Build history of the part. All positions in model axes, mm. A direction names the side the tool comes from. Round coordinates to 2 decimals unless told otherwise and drop trailing zeros. Loops run counter-clockwise (first coordinate to the right, second up) from the corner with the lowest first, then second, coordinate; pieces in that order, holes last. Notation, with made-up numbers: M 25.5,4.25 L 46.5,4.25 A5 ccw 46.5,10.25 Z; hole C 58,-40 d9. An arc over 180 degrees is marked long. Write each question's results on one line, items separated by ' | '. Start each with the question number.
```python
from build123d import *

# Parameters (mm, degrees)
F0_W     = 203.2
F0_H     = 208.396926
F1_DEPTH = 25.4
F2_R     = 25.4
F3_DEPTH = 25.4
F4_R     = 25.4
F5_DEPTH = 25.4


with BuildPart() as f1:
    # F0 (on Top) → F1 (new body)
    with BuildSketch(Plane.XY):
        Rectangle(F0_W, F0_H)
    extrude(amount=F1_DEPTH)

    # F2 (on face) → F3 (join)
    with BuildSketch(Plane.XY.offset(25.4)):
        with Locations((0, 63.5)):
            Circle(F2_R)
    extrude(amount=F3_DEPTH)

    # F4 (on face) → F5 (join, through all)
    with BuildSketch(Plane.XY.offset(25.4)):
        with Locations((0, -70.358)):
            Circle(F4_R)
    extrude(amount=F5_DEPTH)


solid = f1.part
```
Item 1: Saw through at A-A, the plane y = 63.5. Give the cut face in (x, z), then the cut area to 3 significant figures.
Item 2: Drill centre lines: line 1 along Y through (x, z) = (0.5, 39); line 2 along Z through (x, y) = (18.5, 6.5); line 3 along X through (y, z) = (-69, 43.5). Where is each one in solid material? Low to high. Write a range as [from, to].
Item 3: Saw through at B-B, the plane x = 0. Give the cut face in (y, z), then the cut area to 3 significant figures.
Item 4: Saw through at C-C, the plane z = 33.5. Give the cut face in (x, y), then the cut area to 3 significant figures.
Item 5: Drop flat-ended pins along their axis: pin 1 (1 mm diameter, centred on y = 51, z = 34.5, fed in from +X); pin 2 (12 mm diameter, centred on x = -69.5, y = -80, fed in from +Z). Give the stop position or say it passes through.
Item 6: Tool access for faces 5 (the flat face through (0, -70, 50.8)), 6 (the flat face through (-1, 1, 25.4)): list every direction of +Z, -Z, +X, -X, +Y, -Y with a clear straight run to the whole face (end or side of a thin tool).
Item 7: Saw through at D-D, the plane y = -74. Give the cut face in (x, z), then the cut area to 3 significant figures.
Item 8: Mould opens along Y. For faces 1 (the flat face through (-1, 1, 0)), 2 (the cylindrical face through (-5.506, -95.154, 37.922)), 3 (the cylindrical face through (-5.506, 38.704, 37.922)), 4 (the flat face through (-1, -104.198, 13)) say: released by +Y, released by -Y, zero draft, split by the parting line, or undercut.
Working result:
1) outline: M -101.6,0 L 101.6,0 L 101.6,25.4 L 25.4,25.4 L 25.4,50.8 L -25.4,50.8 L -25.4,25.4 L -101.6,25.4 Z | area: 6,450 mm²
2) line 1: y = [-95.75, -44.96], [38.1, 88.9] | line 2: z = [0, 25.4] | line 3: x = [-25.36, 25.36]
3) outline: M -104.2,0 L 104.2,0 L 104.2,25.4 L 88.9,25.4 L 88.9,50.8 L 38.1,50.8 L 38.1,25.4 L -44.96,25.4 L -44.96,50.8 L -95.76,50.8 L -95.76,25.4 L -104.2,25.4 Z | area: 7,870 mm²
4) outline: C 0,-70.36 d50.8; C 0,63.5 d50.8 | area: 4,050 mm²
5) pin 1: stops at x = 22.39 | pin 2: stops at z = 25.4
6) face 5: +Z, +X, -X, +Y, -Y | face 6: +Z
7) outline: M -101.6,0 L 101.6,0 L 101.6,25.4 L 25.14,25.4 L 25.14,50.8 L -25.14,50.8 L -25.14,25.4 L -101.6,25.4 Z | area: 6,440 mm²
8) face 1: zero draft | face 2: undercut | face 3: undercut | face 4: released by -Y
